Source: CAD feature listing. Evaluate the final solid. Frame: model axes, mm. A direction names the side the tool comes from. Give positions to 0.01 mm unless a question says otherwise; leave off trailing zeros. Write each loop counter-clockwise with the first axis right and the second up, starting at its lowest first coordinate (ties: lowest second). Pieces come first, ordered by that corner, then holes. Notation, with made-up numbers: (40, 25) -> (91, 25) arc R11 cw to (91, 30) -> close; hole circle Ø11 at (62, 25.25). An arc over 180 degrees is marked (long way). Write item = value, one per line.
from build123d import *

# Parameters (mm, degrees)
BOSS_EXTRUDE1_DEPTH = 20
SKETCH2_W           = 10
SKETCH2_H           = 27.8
CUT_EXTRUDE1_DEPTH  = 61.882181301
SKETCH4_R           = 11.25
CUT_EXTRUDE3_DEPTH  = 6
SKETCH5_R           = 5.5
CUT_EXTRUDE4_DEPTH  = 1
CUT_EXTRUDE5_DEPTH  = 41.976700697
SKETCH7_R           = 2.6
CUT_EXTRUDE6_DEPTH  = 41.976700765
CUT_EXTRUDE7_DEPTH  = 44.449856262
FILLET1_R           = 4


with BuildPart() as part:
    # Sketch1 → Boss-Extrude1 (new body)
    with BuildSketch(Plane.XY):
        with BuildLine():
            Line((0, 0), (22.5, 0))
            Line((22.5, 0), (22.5, 19))
            Line((22.5, 19), (16.8, 19))
            ThreePointArc((16.8, 19), (0, 35.8), (-16.8, 19))
            Line((-16.8, 19), (-22.5, 19))
            Line((-22.5, 19), (-22.5, 0))
            Line((-22.5, 0), (0, 0))
        make_face()
    extrude(amount=BOSS_EXTRUDE1_DEPTH)

    # Sketch2 → Cut-Extrude1 (cut, through all)
    with BuildSketch(Plane(origin=(22.5, 0, 0), x_dir=(0, 0, -1), z_dir=(1, 0, 0))):
        with Locations((-15, 21.9)):
            Rectangle(SKETCH2_W, SKETCH2_H)
    extrude(amount=-CUT_EXTRUDE1_DEPTH, mode=Mode.SUBTRACT)

    # Sketch4 → Cut-Extrude3 (cut)
    with BuildSketch(Plane.XY.offset(10)):
        with Locations((0, 19)):
            Circle(SKETCH4_R)
    extrude(amount=-CUT_EXTRUDE3_DEPTH, mode=Mode.SUBTRACT)

    # Sketch5 → Cut-Extrude4 (cut)
    with BuildSketch(Plane.XY.offset(4)):
        with Locations((0, 19)):
            Circle(SKETCH5_R)
    extrude(amount=-CUT_EXTRUDE4_DEPTH, mode=Mode.SUBTRACT)

    # Sketch6 → Cut-Extrude5 (cut, through all)
    with BuildSketch(Plane(origin=(0, 8, 0), x_dir=(1, 0, 0), z_dir=(0, 1, 0))):
        with BuildLine():
            Line((-17.5, -5), (-22.5, -5))
            Line((-22.5, -5), (-22.5, -10))
            Line((-22.5, -10), (-12.5, -10))
            ThreePointArc((-12.5, -10), (-13.964466094, -6.464466094), (-17.5, -5))
        make_face()
        with BuildLine():
            Line((17.5, -5), (22.5, -5))
            Line((22.5, -5), (22.5, -10))
            Line((22.5, -10), (12.5, -10))
            ThreePointArc((12.5, -10), (13.964466094, -6.464466094), (17.5, -5))
        make_face()
    extrude(amount=CUT_EXTRUDE5_DEPTH, mode=Mode.SUBTRACT)

    # Sketch7 → Cut-Extrude6 (cut, through all)
    with BuildSketch(Plane(origin=(0, 8, 0), x_dir=(1, 0, 0), z_dir=(0, 1, 0))):
        with Locations(Location((-17.5, -10, 0), (0, 0, 270))):
            Circle(SKETCH7_R)
        with Locations(Location((17.5, -10, 0), (0, 0, 270))):
            Circle(SKETCH7_R)
    extrude(amount=-CUT_EXTRUDE6_DEPTH, mode=Mode.SUBTRACT)

    # Sketch8 → Cut-Extrude7 (cut, through all)
    with BuildSketch(Plane.XY.offset(10)):
        with BuildLine():
            Line((-12.5, 8), (12.5, 8))
            ThreePointArc((12.5, 8), (0, 2.349174195), (-12.5, 8))
        make_face()
    extrude(amount=CUT_EXTRUDE7_DEPTH, mode=Mode.SUBTRACT)

    # Fillet1
    fillet1_edges = [part.edges().sort_by_distance(p)[0] for p in [
        (16.8, 19, 2.524621241),
        (-16.8, 19, 2.524621241),
    ]]
    fillet(fillet1_edges, radius=FILLET1_R)


solid = part.part
1) Cut plane A-A (z = 8). Return the cut outline in (x, y).
Computed:
outline = (-22.5, 0) -> (-19.16, 0) -> (-19.16, 8) -> (-22.5, 8) -> close; (-15.84, 0) -> (15.84, 0) -> (15.84, 8) -> (12.92, 8) -> (12.92, 29.74) arc R16.8 ccw to (-12.92, 29.74) -> (-12.92, 8) -> (-15.84, 8) -> close; (19.16, 0) -> (22.5, 0) -> (22.5, 8) -> (19.16, 8) -> close; hole circle Ø22.5 at (0, 19)
2) Contact query for flat-ended pins moving along their axis: pin 1 (12 mm diameter, centred on x = -14.5, z = 4.5, fed in from +Y); pin 2 (2 mm diameter, centred on x = 4, z = 5, fed in from -Y); pin 3 (1 mm diameter, centred on x = -22, z = 2, fed in from +Y); pin 4 (7.5 mm diameter, centred on x = -5.5, y = 19, fed in from +Z). Output: stop coordinate, or through.
Computed:
pin_1 = 33.49
pin_2 = 0
pin_3 = 19
pin_4 = 4
3) Material intervals for L1, parallel to Y at x = 0, z = 3.55; L2, parallel to Y at x = -17, z = 15.75; L3, parallel to Z at x = -10.5, y = 27.5, sorted ascending.
Computed:
L1 = 0 to 13.5, 24.5 to 35.8
L2 = 0 to 8
L3 = 0 to 10
4) Draft query along Z for faces 6 (the cylindrical face through (-16.72, 4.06, 12.48)), 7 (the flat face through (9, 11, 10)), 8 (the flat face through (0, 14, 0)), 9 (the cylindrical face through (0.2, 2.35, 14.93)). Return one class per face: pulls with the +Z half, pulls with the -Z half, needs draft (parallel to the pull), parting line crosses it, or undercut.
Computed:
face_6 = undercut
face_7 = pulls with the +Z half
face_8 = pulls with the -Z half
face_9 = needs draft
5) Cut plane B-B (x = 19). Return the cut outline in (y, z), then the cut area to 3 significant figures.
Computed:
outline = (0, 0) -> (19.26, 0) -> (19.26, 5) -> (8, 5) -> (8, 7.88) -> (0, 7.88) -> close; (0, 12.12) -> (8, 12.12) -> (8, 20) -> (0, 20) -> close
area = 182 mm²
6) Cut plane D-D (y = 11.5). Return the cut outline in (x, z).
Computed:
outline = (-22.5, 0) -> (22.5, 0) -> (22.5, 5) -> (17.5, 5) arc R5 cw to (12.5, 10) -> (8.39, 10) -> (8.39, 4) -> (-8.39, 4) -> (-8.39, 10) -> (-12.5, 10) arc R5 cw to (-17.5, 5) -> (-22.5, 5) -> close
7) Cut plane C-C (x = 0). Return the cut outline in (y, z).
Computed:
outline = (0, 0) -> (35.8, 0) -> (35.8, 10) -> (30.25, 10) -> (30.25, 4) -> (24.5, 4) -> (24.5, 3) -> (13.5, 3) -> (13.5, 4) -> (7.75, 4) -> (7.75, 10) -> (2.35, 10) -> (2.35, 20) -> (0, 20) -> close
8) Access query for faces 1 (the flat face through (-21, 19, 2)), 2 (the flat face through (-17, 8, 14)), 3 (the flat face through (-22.5, 5, 8)), 4 (the flat face through (20, 14, 5)), 5 (the cylindrical face through (5.19, 9.02, 7.04)). Directions: +Z, -Z, +X, -X, +Y, -Y. A direction counts if a zero-diameter tool reaches every point of the face in a straight line with its end or side. Return the directions, or none.
Computed:
face_1 = +Z, -Z, -X, +Y
face_2 = +Z, -X, +Y
face_3 = +Z, -Z, -X, +Y, -Y
face_4 = +Z, +X, +Y
face_5 = +Z
